The model under review builds one solid part; all positions refer to its coordinate system, in mm. Face numbers are marked on the shaded views. A direction names the side the tool comes from. Coordinates: 2 decimals unless noted, no trailing zeros. Order: outer loops, then holes, each group sorted by start corner. A loop starts at its lowest first (then second) coordinate and runs counter-clockwise, first axis right, second up. Notation, with made-up numbers: M 14.25,20.25 L 20.25,20.25 A12 cw 20.25,40.25 Z; hole C -16,18 d5. An arc over 180 degrees is marked long. One line per item, written item: value.
```python
from build123d import *

# Parameters (mm, degrees)
SALIENTE_EXTRUIR1_DEPTH = 25
SALIENTE_EXTRUIR2_START = -3
SALIENTE_EXTRUIR2_DEPTH = 3
CORTAR_EXTRUIR1_DEPTH   = 3
CROQUIS4_R              = 5.5
CORTAR_EXTRUIR2_DEPTH   = 3


with BuildPart() as part:
    # Croquis1 → Saliente-Extruir1 (new body)
    with BuildSketch(Plane.XY):
        with BuildLine():
            Line((41.445702238, 24.048980806), (60.914091522, 19.468389284))
            ThreePointArc((60.914091522, 19.468389284), (76.3335, 0), (60.914091522, -19.468389284))
            Line((60.914091522, -19.468389284), (41.445702238, -24.048980806))
            ThreePointArc((41.445702238, -24.048980806), (39.191168738, -25.031281724), (37.426574478, -26.744186711))
            ThreePointArc((37.426574478, -26.744186711), (-46, 2.97e-07), (37.426574823, 26.744186228))
            ThreePointArc((37.426574823, 26.744186228), (39.191168984, 25.031281559), (41.445702238, 24.048980806))
        make_face()
        with BuildLine():
            Line((40.758613509, 21.128722413), (60.227002793, 16.548130891))
            ThreePointArc((60.227002793, 16.548130891), (73.3335, 0), (60.227002793, -16.548130891))
            Line((60.227002793, -16.548130891), (40.758613509, -21.128722413))
            ThreePointArc((40.758613509, -21.128722413), (37.520298481, -22.539657237), (34.985711121, -25.000000347))
            ThreePointArc((34.985711121, -25.000000347), (-43, 4.27e-07), (34.985711617, 24.999999653))
            ThreePointArc((34.985711617, 24.999999653), (37.520298835, 22.539656999), (40.758613509, 21.128722413))
        make_face(mode=Mode.SUBTRACT)
    extrude(amount=SALIENTE_EXTRUIR1_DEPTH)

    # Croquis2 → Saliente-Extruir2 (add)
    with BuildSketch(Plane.XY.offset(25).offset(SALIENTE_EXTRUIR2_START)):
        with BuildLine():
            Line((41.445702238, -24.048980806), (60.914091522, -19.468389284))
            ThreePointArc((60.914091522, -19.468389284), (76.3335, 0), (60.914091522, 19.468389284))
            Line((60.914091522, 19.468389284), (41.445702238, 24.048980806))
            ThreePointArc((41.445702238, 24.048980806), (39.191168984, 25.031281559), (37.426574823, 26.744186228))
            ThreePointArc((37.426574823, 26.744186228), (-46, 2.97e-07), (37.426574478, -26.744186711))
            ThreePointArc((37.426574478, -26.744186711), (39.191168738, -25.031281724), (41.445702238, -24.048980806))
        make_face()
    extrude(amount=SALIENTE_EXTRUIR2_DEPTH)

    # Croquis3 → Cortar-Extruir1 (cut)
    with BuildSketch(Plane.XY.offset(25)):
        with BuildLine():
            ThreePointArc((-23.947692308, -34.562794151), (-24.349, -33.76181505), (-23.947692308, -32.960835948))
            ThreePointArc((-23.947692308, -32.960835948), (0, -25), (23.947692308, -32.960835948))
            ThreePointArc((23.947692308, -32.960835948), (24.349, -33.76181505), (23.947692308, -34.562794151))
            ThreePointArc((23.947692308, -34.562794151), (0, -42.523630099), (-23.947692308, -34.562794151))
        make_face()
    extrude(amount=-CORTAR_EXTRUIR1_DEPTH, mode=Mode.SUBTRACT)

    # Croquis4 → Cortar-Extruir2 (cut)
    with BuildSketch(Plane.XY.offset(25)):
        with Locations((56.3335, 0)):
            Circle(CROQUIS4_R)
    extrude(amount=-CORTAR_EXTRUIR2_DEPTH, mode=Mode.SUBTRACT)


solid = part.part
```
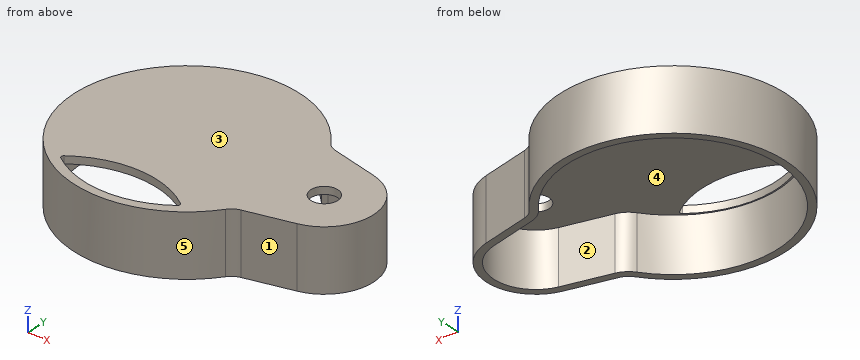
(1) We need section D-D, the plane y = 33.5. State the section outline as (x, z) points.
Geometry results:
outline: M -31.52,0 L -26.96,0 L -26.96,22 L 26.96,22 L 26.96,0 L 31.52,0 L 31.52,25 L -31.52,25 Z
(2) For L1, parallel to Y at x = 0, z = 16.5; L2, parallel to Z at x = -33, y = -15; L3, parallel to X at y = 30, z = 21.25, list the stretches that pass through material, from the lowest coordinate up.
Geometry results:
L1: y = -46 to -43, 43 to 46
L2: z = 22 to 25
L3: x = -34.87 to -30.81, 30.81 to 34.87
(3) We need section B-B, the plane x = 0. State the section outline as (y, z) points.
Geometry results:
outline: M -46,0 L -43,0 L -43,22 L -42.52,22 L -42.52,25 L -46,25 Z; M -25,22 L 43,22 L 43,0 L 46,0 L 46,25 L -25,25 Z
(4) We need section C-C, the plane z = 5.25. State the section outline as (x, y) points, plus the area to 3 significant figures.
Geometry results:
outline: M 37.43,-26.74 A6.88 cw 41.45,-24.05 L 60.91,-19.47 A20 ccw 60.91,19.47 L 41.45,24.05 A6.88 cw 37.43,26.74 A46 ccw long Z; hole M 34.99,-25 A9.88 cw 40.76,-21.13 L 60.23,-16.55 A17 ccw 60.23,16.55 L 40.76,21.13 A9.88 cw 34.99,25 A43 ccw long Z
area: 978 mm2
(5) Insertion check: pin 1 Ø3 at (y, z) = (-32, 19.5) entering from +X; pin 2 Ø4 at (x, z) = (52, 19) entering from -Y; pin 3 Ø8 at (x, z) = (31.5, 16.5) entering from +Y. Each pin has a flat end and moves straight along its axis. Give the tip position at first contact, or say it passes through.
Geometry results:
pin 1: stops at x = 34.43
pin 2: stops at y = -22.04
pin 3: stops at y = 36.87
(6) We need section A-A, the plane y = 0. State the section outline as (x, z) points, plus the area to 3 significant figures.
Geometry results:
outline: M -46,0 L -43,0 L -43,22 L 50.83,22 L 50.83,25 L -46,25 Z; M 61.83,22 L 73.33,22 L 73.33,0 L 76.33,0 L 76.33,25 L 61.83,25 Z
area: 466 mm2
(7) Mouldability with a two-part tool opening along Y and no side actions: class the marked faces 3, 4 and 5 as +Y half, -Y half, draft (parallel to the pull), parting line (faces both ways), or undercut.
Geometry results:
face 3: draft
face 4: undercut
face 5: parting line
(8) Tool access review of the marked faces 1 and 2: name each direction out of +Z, -Z, +X, -X, +Y, -Y from which nothing blocks a thin tool from reaching the whole face with its end or side.
Geometry results:
face 1: +Z, -Z, +X, -Y
face 2: -Z
